from build123d import *

# Parameters (mm, degrees)
SKETCH_R        = 32.5
PAD_DEPTH       = 1
SKETCH001_R     = 27
PAD001_DEPTH    = 3
SKETCH002_R     = 0.95
POCKET_DEPTH    = 5
SKETCH003_R     = 20
POCKET001_DEPTH = 5
FILLET_R        = 1


with BuildPart() as part:
    # Sketch → Pad (new body)
    with BuildSketch(Plane.XY):
        Circle(SKETCH_R)
    extrude(amount=PAD_DEPTH)

    # Sketch001 (on Face3 of Pad) → Pad001 (join)
    with BuildSketch(Plane.XY.offset(1)):
        Circle(SKETCH001_R)
    extrude(amount=PAD001_DEPTH)

    # Sketch002 (on Face5 of Pad001) → Pocket (cut)
    with BuildSketch(Plane.XY.offset(4)):
        with Locations((-16, 16)):
            Circle(SKETCH002_R)
        with Locations((16, 16)):
            Circle(SKETCH002_R)
        with Locations((-16, -16)):
            Circle(SKETCH002_R)
        with Locations((16, -16)):
            Circle(SKETCH002_R)
    extrude(amount=-POCKET_DEPTH, mode=Mode.SUBTRACT)

    # Sketch003 (on Face9 of Pocket) → Pocket001 (cut)
    with BuildSketch(Plane.XY.offset(4)):
        Circle(SKETCH003_R)
        with BuildLine():
            ThreePointArc((10, 25.079872408), (0, 27), (-10, 25.079872408))
            Line((-12.037037037, 30.1887353059), (-10, 25.079872408))
            ThreePointArc((12.037037037, 30.1887353059), (0, 32.5), (-12.037037037, 30.1887353059))
            Line((10, 25.079872408), (12.037037037, 30.1887353059))
        make_face()
    extrude(amount=-POCKET001_DEPTH, mode=Mode.SUBTRACT)

    # Fillet
    fillet_edges = [part.edges().sort_by_distance(p)[0] for p in [
        (12.037037, 30.188735, 0.5),
        (-12.037037, 30.188735, 0.5),
        (-10, 25.079872, 0.5),
        (10, 25.079872, 0.5),
    ]]
    fillet(fillet_edges, radius=FILLET_R)


solid = part.part
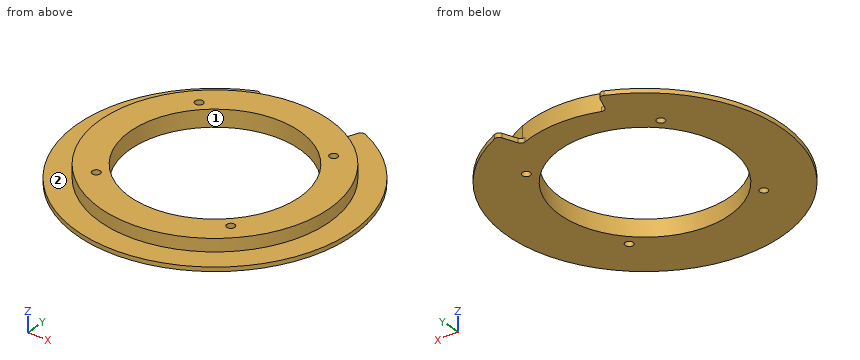
CAD build for the part. Positions are in the model's coordinates, mm. Face numbers are marked on the shaded views. Round coordinates to 2 decimals unless told otherwise and drop trailing zeros. Write each loop counter-clockwise with the first axis right and the second up, starting at its lowest first coordinate (ties: lowest second). Pieces come first, ordered by that corner, then holes. Notation, with made-up numbers: M 21,28 L 74,28 A30 cw 74,54 Z; hole C 43.5,17 d2. An arc over 180 degrees is marked long. Use a Markdown table: item, result. Add a question column.
1. Slice it at A-A on x = 0. Give the cut face in (y, z).
2. Drill centre lines: probe 1 along Y at (x, z) = (16, 0.9); probe 2 along Y at (x, z) = (16, 2.2); probe 3 along Z at (x, y) = (21, 17.5). Where is each one in solid material? Low to high.
3. Slice it at B-B on y = 0. Give the cut face in (x, z).
4. Slice it at D-D on y = -16. Give the cut face in (x, z), then the cut area to 3 significant figures.
5. Slice it at C-C on z = 3. Give the cut face in (x, y).
6. Pull direction Y, two halves, no side cores. Call the marked faces 1 and 2: released by +Y, released by -Y, zero draft, split by the parting line, or undercut.
Reply:
| question | item | result |
|---|---|---|
| 1 | outline | M -32.5,0 L -20,0 L -20,4 L -27,4 L -27,1 L -32.5,1 Z; M 20,0 L 27,0 L 27,4 L 20,4 Z |
| 2 | probe 1 | y = -28.29 to -16.95, -15.05 to -12, 12 to 15.05, 16.95 to 28.29 |
| 2 | probe 2 | y = -21.75 to -16.95, -15.05 to -12, 12 to 15.05, 16.95 to 21.75 |
| 2 | probe 3 | z = 0 to 1 |
| 3 | outline | M -32.5,0 L -20,0 L -20,4 L -27,4 L -27,1 L -32.5,1 Z; M 20,0 L 32.5,0 L 32.5,1 L 27,1 L 27,4 L 20,4 Z |
| 4 | outline | M -28.29,0 L -16.95,0 L -16.95,4 L -21.75,4 L -21.75,1 L -28.29,1 Z; M -15.05,0 L -12,0 L -12,4 L -15.05,4 Z; M 12,0 L 15.05,0 L 15.05,4 L 12,4 Z; M 16.95,0 L 28.29,0 L 28.29,1 L 21.75,1 L 21.75,4 L 16.95,4 Z |
| 4 | area | 75.9 mm^2 |
| 5 | outline | C 0,0 d54; hole C 0,0 d40; hole C -16,-16 d1.9; hole C -16,16 d1.9; hole C 16,-16 d1.9; hole C 16,16 d1.9 |
| 6 | face 1 | undercut |
| 6 | face 2 | zero draft |
